from build123d import *

# Parameters (mm, degrees)
RESSALTO_EXTRUS_O2_OUTLINE_W = 30
RESSALTO_EXTRUS_O2_OUTLINE_H = 24
RESSALTO_EXTRUS_O2_OUTLINE_R = 1.5
RESSALTO_EXTRUS_O2_DEPTH     = 3
ESBO_O5_W                    = 30
ESBO_O5_H                    = 10
CORTE_EXTRUS_O2_DEPTH        = 1
RESSALTO_EXTRUS_O3_START     = -3.000012
ESBO_O6_R                    = 2
ESBO_O6_R_2                  = 1.75
RESSALTO_EXTRUS_O3_DEPTH     = 5.000012


# Read off the part's stored shape, not the designer's step: Ressalto-extrusão2
with BuildPart() as part:
    # Ressalto-extrusão2 outline → Ressalto-extrusão2 (new body)
    with BuildSketch(Plane.XY):
        with Locations((0, 10.5)):
            Rectangle(RESSALTO_EXTRUS_O2_OUTLINE_W, RESSALTO_EXTRUS_O2_OUTLINE_H)
        with Locations((12, 4.5)):
            Circle(RESSALTO_EXTRUS_O2_OUTLINE_R, mode=Mode.SUBTRACT)
        with Locations((-12.5, 19.897915762)):
            Circle(RESSALTO_EXTRUS_O2_OUTLINE_R, mode=Mode.SUBTRACT)
        with Locations((-7, 17.5)):
            Circle(RESSALTO_EXTRUS_O2_OUTLINE_R, mode=Mode.SUBTRACT)
        with Locations((7, 17.5)):
            Circle(RESSALTO_EXTRUS_O2_OUTLINE_R, mode=Mode.SUBTRACT)
        with Locations((12.5, 19.897915762)):
            Circle(RESSALTO_EXTRUS_O2_OUTLINE_R, mode=Mode.SUBTRACT)
    extrude(amount=RESSALTO_EXTRUS_O2_DEPTH)

    # Esboço5 → Corte-extrusão2 (cut)
    with BuildSketch(Plane(origin=(0, 0, 0), x_dir=(-1, 0, 0), z_dir=(0, 0, -1))):
        with Locations((0, 3.5)):
            Rectangle(ESBO_O5_W, ESBO_O5_H)
    extrude(amount=-CORTE_EXTRUS_O2_DEPTH, mode=Mode.SUBTRACT)

    # Esboço6 → Ressalto-extrusão3 (add)
    with BuildSketch(Plane(origin=(0, 0, 0), x_dir=(-1, 0, 0), z_dir=(0, 0, -1)).offset(RESSALTO_EXTRUS_O3_START)):
        Polygon((-15, 8.5), (15, 8.5), (15, 32.5), (6, 32.5), (6, 22.5), (-6, 22.5), (-6, 32.5), (-15, 32.5), align=None)
        with Locations((12.5, 19.897915762)):
            Circle(ESBO_O6_R, mode=Mode.SUBTRACT)
        with Locations((7, 17.5)):
            Circle(ESBO_O6_R, mode=Mode.SUBTRACT)
        with Locations((-7, 17.5)):
            Circle(ESBO_O6_R, mode=Mode.SUBTRACT)
        with Locations((-12.5, 19.897915762)):
            Circle(ESBO_O6_R, mode=Mode.SUBTRACT)
        with Locations((-12.5, 29.5)):
            Circle(ESBO_O6_R_2, mode=Mode.SUBTRACT)
        with Locations((12.5, 29.5)):
            Circle(ESBO_O6_R_2, mode=Mode.SUBTRACT)
    extrude(amount=RESSALTO_EXTRUS_O3_DEPTH)


solid = part.part
Source: CAD feature listing. Evaluate the final solid. Frame: model axes, mm. A direction names the side the tool comes from. Give positions to 0.01 mm unless a question says otherwise; leave off trailing zeros. Write each loop counter-clockwise with the first axis right and the second up, starting at its lowest first coordinate (ties: lowest second). Pieces come first, ordered by that corner, then holes. Notation, with made-up numbers: (-37.5, 47) -> (-31.5, 47) arc R22 cw to (-31.5, 86) -> close; hole circle Ø4 at (50, -33). An arc over 180 degrees is marked (long way). Return JSON: item names as keys, results as strings. Group by question number.
1. Section A-A, the plane y = 29.5. Output: boundary loops of the cut face in (x, z).
2. Access query for faces 1 (the face through (0, 4, 1)), 2 (the face through (8, 19, 0)), 3 (the face through (-6, 28, 1)). Directions: +Z, -Z, +X, -X, +Y, -Y. A direction counts if a zero-diameter tool reaches every point of the face in a straight line with its end or side. Return the directions, or none.
3. Section C-C, the plane y = 17.5. Count the separate pieces of the cut face and the enclosed holes in it, then the cut area to 3 significant figures.
4. Pin query (flat end, axial travel): pin 1 Ø1.5 at (x, z) = (-5.5, -0.5) entering from -Y; pin 2 Ø1.8 at (x, y) = (7, 17.5) entering from -Z. Return the tip coordinate at first contact, or that it passes through.
5. Material intervals for line 1 (X direction, y = 17.5, z = -0.55); line 2 (Y direction, x = 12.5, z = -1.4); line 3 (Y direction, x = 7, z = 0.65), sorted ascending. Write a range as from..to.
Determined:
{
 "1": {"outline": "(-15, -2) -> (-14.25, -2) -> (-14.25, 3) -> (-15, 3) -> close; (-10.75, -2) -> (-6, -2) -> (-6, 3) -> (-10.75, 3) -> close; (6, -2) -> (10.75, -2) -> (10.75, 3) -> (6, 3) -> close; (14.25, -2) -> (15, -2) -> (15, 3) -> (14.25, 3) -> close"},
 "2": {"face 1": "-Z, +X, -X, -Y", "face 2": "-Z", "face 3": "+Z, -Z, +Y"},
 "3": {"separate pieces": "3", "enclosed holes": "0", "area": "116 mm2"},
 "4": {"pin 1": "stops at y = 8.5", "pin 2": "passes through"},
 "5": {"line 1": "x = -15..-9, -5..5, 9..15", "line 2": "y = 8.5..17.9, 21.9..27.75, 31.25..32.5", "line 3": "y = 8.5..16, 19..32.5"}
}
